from build123d import *

# Parameters (mm, degrees)
BOSS_EXTRU_1_DEPTH                                 = 15
CHAMBRAGE_POUR_VIS_T_TE_HEXAGONALE_M31_D           = 3.4
CHAMBRAGE_POUR_VIS_T_TE_HEXAGONALE_M31_CBORE_D     = 6.5
CHAMBRAGE_POUR_VIS_T_TE_HEXAGONALE_M31_CBORE_DEPTH = 3.4
ENL_V_MAT_EXTRU_2_REACH                            = 51.74
ESQUISSE3_W                                        = 10
ESQUISSE3_H                                        = 26.208058997
ESQUISSE2_W                                        = 20.4
ESQUISSE2_H                                        = 20.4
ENL_V_MAT_EXTRU_1_DEPTH                            = 38.791941003
CHAMBRAGE_POUR_VIS_T_TE_HEXAGONALE_M42_D           = 4.5
CHAMBRAGE_POUR_VIS_T_TE_HEXAGONALE_M42_DEPTH       = 4.8
CHAMBRAGE_POUR_VIS_T_TE_HEXAGONALE_M42_CBORE_D     = 8
CHAMBRAGE_POUR_VIS_T_TE_HEXAGONALE_M42_CBORE_DEPTH = 1
CHAMBRAGE_POUR_VIS_T_TE_HEXAGONALE_M43_D           = 4.5
CHAMBRAGE_POUR_VIS_T_TE_HEXAGONALE_M43_CBORE_D     = 8
CHAMBRAGE_POUR_VIS_T_TE_HEXAGONALE_M43_CBORE_DEPTH = 4.4


with BuildPart() as part:
    # Esquisse1 → Boss.-Extru.1 (new, symmetric)
    with BuildSketch(Plane(origin=(0, 0, 0), x_dir=(0, 0, -1), z_dir=(1, 0, 0))):
        with BuildLine():
            Line((-12.5, -40.299852287), (-12.5, 17.200147713))
            ThreePointArc((-12.5, 17.200147713), (0, 29.700147713), (12.5, 17.200147713))
            Line((12.5, 17.200147713), (12.5, -40.299852287))
            Line((12.5, -40.299852287), (-12.5, -40.299852287))
        make_face()
    extrude(amount=BOSS_EXTRU_1_DEPTH, both=True)

    # Chambrage pour vis à tête hexagonale M31 (through all)
    with Locations(Plane(origin=(15, 0, 0), x_dir=(0, 0, -1), z_dir=(1, 0, 0))):
        with Locations((0, 17.200147713)):
            CounterBoreHole(CHAMBRAGE_POUR_VIS_T_TE_HEXAGONALE_M31_D / 2, CHAMBRAGE_POUR_VIS_T_TE_HEXAGONALE_M31_CBORE_D / 2, CHAMBRAGE_POUR_VIS_T_TE_HEXAGONALE_M31_CBORE_DEPTH)

    # Esquisse3 → Enlèv. mat.-Extru.2 (cut, up to next)
    with BuildSketch(Plane(origin=(0, 0, -12.5), x_dir=(-1, 0, 0), z_dir=(0, 0, -1)), mode=Mode.PRIVATE) as enl_v_mat_extru_2_sk1:
        with Locations((0, 16.596118215)):
            Rectangle(ESQUISSE3_W, ESQUISSE3_H)
    enl_v_mat_extru_2_tool1 = extrude(enl_v_mat_extru_2_sk1.sketch, amount=-ENL_V_MAT_EXTRU_2_REACH, mode=Mode.PRIVATE) & part.part
    add(enl_v_mat_extru_2_tool1.solids().sort_by_distance((0, 16.596118, -12.5))[0], mode=Mode.SUBTRACT)

    # Esquisse2 → Enlèv. mat.-Extru.1 (cut)
    with BuildSketch(Plane.XZ.offset(40.299852287)):
        Rectangle(ESQUISSE2_W, ESQUISSE2_H)
    extrude(amount=-ENL_V_MAT_EXTRU_1_DEPTH, mode=Mode.SUBTRACT)

    # Chambrage pour vis à tête hexagonale M42
    with Locations(Plane.ZY.offset(15)):
        with Locations((0, -18.495042181)):
            chambrage_pour_vis_t_te_hexagonale_m42 = CounterBoreHole(CHAMBRAGE_POUR_VIS_T_TE_HEXAGONALE_M42_D / 2, CHAMBRAGE_POUR_VIS_T_TE_HEXAGONALE_M42_CBORE_D / 2, CHAMBRAGE_POUR_VIS_T_TE_HEXAGONALE_M42_CBORE_DEPTH, depth=CHAMBRAGE_POUR_VIS_T_TE_HEXAGONALE_M42_DEPTH)

    # Chambrage pour vis à tête hexagonale M43 (through all)
    with Locations(Plane(origin=(0, 3.492088716, 0), x_dir=(1, 0, 0), z_dir=(0, 1, 0))):
        with Locations((0, 0)):
            CounterBoreHole(CHAMBRAGE_POUR_VIS_T_TE_HEXAGONALE_M43_D / 2, CHAMBRAGE_POUR_VIS_T_TE_HEXAGONALE_M43_CBORE_D / 2, CHAMBRAGE_POUR_VIS_T_TE_HEXAGONALE_M43_CBORE_DEPTH)

    # Symétrie1: Chambrage pour vis à tête hexagonale M42 across plane
    add(chambrage_pour_vis_t_te_hexagonale_m42.mirror(Plane(origin=(0, 0, 0), x_dir=(0, 0, 1), z_dir=(1, 0, 0))), mode=Mode.SUBTRACT)


solid = part.part
Input: part model. Units: mm. Frame: model coordinates. A direction names the side the tool comes from. Give positions to 0.01 mm unless a question says otherwise; leave off trailing zeros. Write each loop counter-clockwise with the first axis right and the second up, starting at its lowest first coordinate (ties: lowest second). Pieces come first, ordered by that corner, then holes. Notation, with made-up numbers: M 26,41 L 77,41 A22 cw 77,59 Z; hole C 16.25,45 d8. An arc over 180 degrees is marked long. Use one line per item in the form item = value.
1. Mould query, pull axis Z, two halves, no side actions, for faces 4 (the face through (8.25, 15.54, -0.37)), 5 (the face through (-5, 14, 0)), 6 (the face through (0, -11, -12.5)). Classes: released by +Z, released by -Z, zero draft, split by the parting line, or undercut.
Outcome:
face_4 = undercut
face_5 = zero draft
face_6 = released by -Z
2. First-contact query: P1, Ø7, axis at y = -18.5, z = 0, coming from the -X side; P2, Ø2, axis at x = -7, z = 7, coming from the -Y side; P3, Ø9, axis at x = 0, z = 0, coming from the +Y side. Flat tips, straight axial feed; report the tip coordinate or a pass-through.
Outcome:
P1 = -14
P2 = -1.51
P3 = 3.49
3. Ray query, L1, parallel to Y at x = -11.6, z = 0; L2, parallel to Y at x = -7.5, z = 0; L3, parallel to X at y = -3.5, z = 5. Return the intervals inside material, ascending.
Outcome:
L1 = -40.3 to -20.75, -16.25 to 15.5, 18.9 to 29.7
L2 = -1.51 to 15.5, 18.9 to 29.7
L3 = -15 to -10.2, 10.2 to 15
4. Reachability of faces 1 (the face through (0, -21, -10.2)), 2 (the face through (14.51, -22.04, 1.85)), 3 (the face through (5, 14, 0)) from +Z, -Z, +X, -X, +Y, -Y: full face, straight path, thin tool, end or side. Return the list, or none.
Outcome:
face_1 = -Y
face_2 = +X
face_3 = +Z, -Z, +Y
5. Cut plane D-D on y = 21.5. Return loops of the section in (x, z), and give its area (3 significant figures).
Outcome:
outline = M -15,-11.74 L -5,-11.74 L -5,11.74 L -15,11.74 Z; M 5,-11.74 L 15,-11.74 L 15,11.74 L 5,11.74 Z
area = 469 mm²
6. Cut plane B-B on x = -5.75. Return loops of the section in (y, z).
Outcome:
outline = M -40.3,-12.5 L 17.2,-12.5 A12.5 ccw 17.2,12.5 L -40.3,12.5 L -40.3,10.2 L -1.51,10.2 L -1.51,-10.2 L -40.3,-10.2 Z; hole C 17.2,0 d3.4
7. Cut plane C-C on y = -31. Return loops of the section in (x, z), and give its area (3 significant figures).
Outcome:
outline = M -15,-12.5 L 15,-12.5 L 15,12.5 L -15,12.5 Z; hole M -10.2,-10.2 L 10.2,-10.2 L 10.2,10.2 L -10.2,10.2 Z
area = 334 mm²
8. Cut plane A-A on x = 0. Return loops of the section in (y, z), and give its area (3 significant figures).
Outcome:
outline = M -40.3,-12.5 L 3.49,-12.5 L 3.49,-4 L -0.91,-4 L -0.91,-2.25 L -1.51,-2.25 L -1.51,-10.2 L -40.3,-10.2 Z; M -40.3,10.2 L -1.51,10.2 L -1.51,2.25 L -0.91,2.25 L -0.91,4 L 3.49,4 L 3.49,12.5 L -40.3,12.5 Z
area = 266 mm²
